from build123d import *

# Parameters (mm, degrees)
F0_R     = 9.525
F1_DEPTH = 19.05
F2_DEPTH = 50.8
F3_DEPTH = 38.1


with BuildPart() as f1:
    # F0 (on Front) → F1 (new body)
    with BuildSketch(Plane.XZ):
        with BuildLine():
            Line((-59.729688, -13.125407), (-25.003125, -36.751139))
            ThreePointArc((-25.003125, -36.751139), (1.727006, -44.416438), (27.78125, -34.69877))
            Line((27.78125, -34.69877), (58.7375, -9.913934))
            ThreePointArc((58.7375, -9.913934), (63.5, 0), (58.7375, 9.913934))
            Line((58.7375, 9.913934), (27.78125, 34.69877))
            ThreePointArc((27.78125, 34.69877), (1.727006, 44.416438), (-25.003125, 36.751139))
            Line((-25.003125, 36.751139), (-59.729688, 13.125407))
            ThreePointArc((-59.729688, 13.125407), (-66.675, 0), (-59.729688, -13.125407))
        make_face()
        with Locations((-50.8, 0)):
            Circle(F0_R, mode=Mode.SUBTRACT)
        with BuildLine():
            ThreePointArc((34.342876, 6.35), (34.779164, 3.188313), (34.925, 0))
            ThreePointArc((34.925, 0), (34.779164, -3.188313), (34.342876, -6.35))
            ThreePointArc((34.342876, -6.35), (24.695704, -24.695704), (6.35, -34.342876))
            ThreePointArc((6.35, -34.342876), (0, -34.925), (-6.35, -34.342876))
            ThreePointArc((-6.35, -34.342876), (-24.695704, -24.695704), (-34.342876, -6.35))
            ThreePointArc((-34.342876, -6.35), (-34.779164, -3.188313), (-34.925, 0))
            ThreePointArc((-34.925, 0), (-34.779164, 3.188313), (-34.342876, 6.35))
            ThreePointArc((-34.342876, 6.35), (-24.695704, 24.695704), (-6.35, 34.342876))
            ThreePointArc((-6.35, 34.342876), (0, 34.925), (6.35, 34.342876))
            ThreePointArc((6.35, 34.342876), (24.695704, 24.695704), (34.342876, 6.35))
        make_face(mode=Mode.SUBTRACT)
        with BuildLine():
            ThreePointArc((57.15, 0), (50.8, -6.35), (44.45, 0))
            ThreePointArc((44.45, 0), (50.8, 6.35), (57.15, 0))
        make_face(mode=Mode.SUBTRACT)
    extrude(amount=F1_DEPTH)

    # F0 (on Front) → F2 (join)
    with BuildSketch(Plane.XZ):
        with BuildLine():
            Line((-34.342876, 6.35), (-24.593444, 6.35))
            ThreePointArc((-24.593444, 6.35), (-17.960512, 17.960512), (-6.35, 24.593444))
            Line((-6.35, 24.593444), (-6.35, 34.342876))
            ThreePointArc((-6.35, 34.342876), (-24.695704, 24.695704), (-34.342876, 6.35))
        make_face()
        with BuildLine():
            ThreePointArc((6.35, 24.593444), (17.960512, 17.960512), (24.593444, 6.35))
            Line((24.593444, 6.35), (34.342876, 6.35))
            ThreePointArc((34.342876, 6.35), (24.695704, 24.695704), (6.35, 34.342876))
            Line((6.35, 34.342876), (6.35, 24.593444))
        make_face()
        with BuildLine():
            Line((34.342876, -6.35), (24.593444, -6.35))
            ThreePointArc((24.593444, -6.35), (17.960512, -17.960512), (6.35, -24.593444))
            Line((6.35, -24.593444), (6.35, -34.342876))
            ThreePointArc((6.35, -34.342876), (24.695704, -24.695704), (34.342876, -6.35))
        make_face()
        with BuildLine():
            ThreePointArc((-6.35, -24.593444), (-17.960512, -17.960512), (-24.593444, -6.35))
            Line((-24.593444, -6.35), (-34.342876, -6.35))
            ThreePointArc((-34.342876, -6.35), (-24.695704, -24.695704), (-6.35, -34.342876))
            Line((-6.35, -34.342876), (-6.35, -24.593444))
        make_face()
    extrude(amount=F2_DEPTH)

    # F0 (on Front) → F3 (join)
    with BuildSketch(Plane.XZ):
        with BuildLine():
            ThreePointArc((-12.7, 0), (0, 12.7), (12.7, 0))
            Line((12.7, 0), (25.4, 0))
            ThreePointArc((25.4, 0), (25.197554, 3.200509), (24.593444, 6.35))
            ThreePointArc((24.593444, 6.35), (17.960512, 17.960512), (6.35, 24.593444))
            ThreePointArc((6.35, 24.593444), (0, 25.4), (-6.35, 24.593444))
            ThreePointArc((-6.35, 24.593444), (-17.960512, 17.960512), (-24.593444, 6.35))
            ThreePointArc((-24.593444, 6.35), (-25.197554, 3.200509), (-25.4, 0))
            Line((-25.4, 0), (-12.7, 0))
        make_face()
        with BuildLine():
            Line((25.4, 0), (12.7, 0))
            ThreePointArc((12.7, 0), (0, -12.7), (-12.7, 0))
            Line((-12.7, 0), (-25.4, 0))
            ThreePointArc((-25.4, 0), (-25.197554, -3.200509), (-24.593444, -6.35))
            ThreePointArc((-24.593444, -6.35), (-17.960512, -17.960512), (-6.35, -24.593444))
            ThreePointArc((-6.35, -24.593444), (0, -25.4), (6.35, -24.593444))
            ThreePointArc((6.35, -24.593444), (17.960512, -17.960512), (24.593444, -6.35))
            ThreePointArc((24.593444, -6.35), (25.197554, -3.200509), (25.4, 0))
        make_face()
    extrude(amount=F3_DEPTH)


solid = f1.part
Geometry check sheet. Reference: the model listing, model coordinates, mm. A direction names the side the tool comes from. Round coordinates to 2 decimals unless told otherwise and drop trailing zeros. Order: outer loops, then holes, each group sorted by start corner. A loop starts at its lowest first (then second) coordinate and runs counter-clockwise, first axis right, second up. Notation, with made-up numbers: M 13.25,52 L 31.25,52 A28 cw 31.25,72 Z; hole C 39,47.25 d3. An arc over 180 degrees is marked long. Answer in a Markdown table with one row per item. Add a question column.
Item 1: Depth check by flat-ended pin: pin 1 Ø3 at (x, y) = (-27.5, -21) entering from -Z; pin 2 Ø8 at (y, z) = (-21, -31) entering from -X; pin 3 Ø4 at (y, z) = (-20.5, 12) entering from -X; pin 4 Ø7.5 at (x, z) = (50.8, 0) entering from +Y. Enter the tip coordinate at first touch or a pass-through.
Item 2: Sectioned sample at B-B, the plane x = 0. Enter the section's corners in (y, z) (3 decimals).
Item 3: Draft check along X on faces 1 (the face through (0.1, -18.8, 25.4)), 2 (the face through (-36, -19.05, -3)), 3 (the face through (44.743, -9.392, 1.907)), 4 (the face through (43.48, -9.39, 22.13)). Enter one of: released by +X, released by -X, zero draft, split by the parting line, or undercut.
Item 4: Sectioned sample at D-D, the plane z = 33. Enter the section's corners in (x, y), plus the area to 3 significant figures.
Item 5: Sectioned sample at A-A, the plane y = -44.5. Enter the section's corners in (x, z) (3 decimals).
Item 6: Set-up check for faces 5 (the face through (24.9, -34.7, 24.49)), 6 (the face through (-30, -25, 6.35)), 7 (the face through (-17.83, -44.36, -18.09)): record each of +Z, -Z, +X, -X, +Y, -Y from which the full face is reachable in a straight line by a thin tool's end or side.
Item 7: Material ranges on L1, parallel to Z at x = 0, y = -9 (3 decimals); L2, parallel to Z at x = 0, y = -21; L3, parallel to Y at x = -58.5, z = 11, recorded low to high. Write a range as [from, to].
Item 8: Sectioned sample at C-C, the plane x = 49. Enter the section's corners in (y, z), plus the area to 3 significant figures.
Filled in:
| question | item | result |
|---|---|---|
| 1 | pin 1 | stops at z = -23.32 |
| 1 | pin 2 | stops at x = -38.59 |
| 1 | pin 3 | stops at x = -62.6 |
| 1 | pin 4 | passes through |
| 2 | outline | M -38.1,-25.4 L 0,-25.4 L 0,-12.7 L -38.1,-12.7 Z; M -38.1,12.7 L 0,12.7 L 0,25.4 L -38.1,25.4 Z; M -19.05,-44.45 L 0,-44.45 L 0,-34.925 L -19.05,-34.925 Z; M -19.05,34.925 L 0,34.925 L 0,44.45 L -19.05,44.45 Z |
| 3 | face 1 | undercut |
| 3 | face 2 | zero draft |
| 3 | face 3 | undercut |
| 3 | face 4 | released by +X |
| 4 | outline | M -30.52,-19.05 L -11.43,-19.05 L -11.43,-50.8 L -6.35,-50.8 L -6.35,0 L -30.52,0 Z; M 6.35,-50.8 L 11.43,-50.8 L 11.43,-19.05 L 29.9,-19.05 L 29.9,0 L 6.35,0 Z |
| 4 | area | 1,230 mm² |
| 5 | outline | M -34.343,-6.35 A34.925 ccw -6.35,-34.343 L -6.35,-24.593 A25.4 cw -24.593,-6.35 Z; M -34.343,6.35 L -24.593,6.35 A25.4 cw -6.35,24.593 L -6.35,34.343 A34.925 ccw Z; M 6.35,-34.343 A34.925 ccw 34.343,-6.35 L 24.593,-6.35 A25.4 cw 6.35,-24.593 Z; M 6.35,24.593 A25.4 cw 24.593,6.35 L 34.343,6.35 A34.925 ccw 6.35,34.343 Z |
| 6 | face 5 | +Z, +X, -Y |
| 6 | face 6 | +Y, -Y |
| 6 | face 7 | -Y |
| 7 | L1 | z = [-44.45, -34.925], [-25.4, -12.7], [12.7, 25.4], [34.925, 44.45] |
| 7 | L2 | z = [-25.4, -12.7], [12.7, 25.4] |
| 7 | L3 | y = [-19.05, 0] |
| 8 | outline | M -19.05,-17.71 L 0,-17.71 L 0,-6.09 L -19.05,-6.09 Z; M -19.05,6.09 L 0,6.09 L 0,17.71 L -19.05,17.71 Z |
| 8 | area | 443 mm² |
